```python
from build123d import *

# Parameters (mm, degrees)
F0_W     = 150
F0_H     = 85
F1_DEPTH = 85
F2_R     = 6.25
F3_DEPTH = 85.001
F2_R_2   = 11.5
F4_DEPTH = 25
F6_D     = 11


with BuildPart() as f1:
    # F0 (on Top) → F1 (new body)
    with BuildSketch(Plane.XY):
        with Locations((75, 42.5)):
            Rectangle(F0_W, F0_H)
    extrude(amount=F1_DEPTH)

    # F2 (on face) → F3 (cut, through all)
    with BuildSketch(Plane.XZ):
        with Locations((75, 63.75)):
            Circle(F2_R)
        with Locations((75, 21.25)):
            Circle(F2_R)
    extrude(amount=-F3_DEPTH, mode=Mode.SUBTRACT)

    # F2 (on face) → F4 (cut)
    with BuildSketch(Plane.XZ):
        with Locations((75, 63.75)):
            Circle(F2_R_2)
        with Locations((75, 63.75)):
            Circle(F2_R, mode=Mode.SUBTRACT)
        with Locations((75, 21.25)):
            Circle(F2_R_2)
        with Locations((75, 21.25)):
            Circle(F2_R, mode=Mode.SUBTRACT)
    extrude(amount=-F4_DEPTH, mode=Mode.SUBTRACT)

    # F6 (through all)
    with Locations(Plane.XY.offset(85)):
        with Locations((20, 65), (20, 20), (130, 20), (130, 65)):
            Hole(F6_D / 2)


solid = f1.part
```
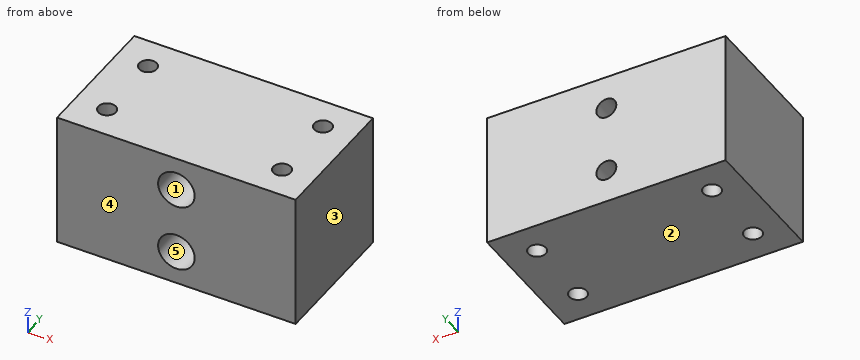
The listing builds one solid part. Answer for the finished solid, in the listing's coordinates (mm). Face numbers are marked on the shaded views. A direction names the side the tool comes from. Coordinates: 2 decimals unless noted, no trailing zeros. Order: outer loops, then holes, each group sorted by start corner. A loop starts at its lowest first (then second) coordinate and runs counter-clockwise, first axis right, second up. Notation, with made-up numbers: M -23,49 L -9,49 A16 cw -9,72 Z; hole C 21.25,32 d9. An arc over 180 degrees is marked long. Answer as a JSON object with one key per item and string values. Group by question number.
1. Section C-C on x = 20 is taken. Write down the section's boundary in (y, z), then the cut area to 4 significant figures.
2. Flat-ended cylindrical pins translate along their axes: P1, Ø8, axis at y = 51, z = 48.5, coming from the -X side; P2, Ø11.5, axis at x = 77, z = 19.5, coming from the -Y side. Find the tip coordinate at first contact, or state that the pin passes through.
3. Determine the mould class of the marked faces 1, 2 and 3 for opening direction Z: released by +Z, released by -Z, zero draft, split by the parting line, or undercut.
4. Section A-A on y = 20 is taken. Write down the section's boundary in (x, z), then the cut area to 3 significant figures.
5. A tool of negligible diameter and unlimited length cuts with its end or side. For the marked faces 4 and 5, from which of +Z, -Z, +X, -X, +Y, -Y can it reach the whole face along a straight path? Write none if from no direction.
6. Straight lines are drawn through the part: line 1 (Z direction, x = 75, y = 61.5); line 2 (X direction, y = 64.5, z = 56); line 3 (Z direction, x = 75, y = 16). For each, find the intervals that lie inside material, in ascending order.
7. Section D-D on y = 37 is taken. Write down the section's boundary in (x, z).
8. Section B-B on z = 21.25 is taken. Write down the section's boundary in (x, y).
Values follow:
{
 "1": {"outline": "M 0,0 L 14.5,0 L 14.5,85 L 0,85 Z; M 25.5,0 L 59.5,0 L 59.5,85 L 25.5,85 Z; M 70.5,0 L 85,0 L 85,85 L 70.5,85 Z", "area": "5,355 mm2"},
 "2": {"P1": "x = 0", "P2": "y = 25"},
 "3": {"face 1": "undercut", "face 2": "released by -Z", "face 3": "zero draft"},
 "4": {"outline": "M 0,0 L 14.5,0 L 14.5,85 L 0,85 Z; M 25.5,0 L 124.5,0 L 124.5,85 L 25.5,85 Z; M 135.5,0 L 150,0 L 150,85 L 135.5,85 Z; hole C 75,21.25 d23; hole C 75,63.75 d23", "area": "10,000 mm2"},
 "5": {"face 4": "+Z, -Z, +X, -X, -Y", "face 5": "-Y"},
 "6": {"line 1": "0 to 15, 27.5 to 57.5, 70 to 85", "line 2": "0 to 14.52, 25.48 to 124.52, 135.48 to 150", "line 3": "0 to 9.75, 32.75 to 52.25, 75.25 to 85"},
 "7": {"outline": "M 0,0 L 150,0 L 150,85 L 0,85 Z; hole C 75,21.25 d12.5; hole C 75,63.75 d12.5"},
 "8": {"outline": "M 0,0 L 63.5,0 L 63.5,25 L 68.75,25 L 68.75,85 L 0,85 Z; M 81.25,25 L 86.5,25 L 86.5,0 L 150,0 L 150,85 L 81.25,85 Z; hole C 20,20 d11; hole C 20,65 d11; hole C 130,20 d11; hole C 130,65 d11"}
}
